Geometry: final body of the model. Coordinates: model frame, mm. A direction names the side the tool comes from. Give positions to 0.01 mm unless a question says otherwise; leave off trailing zeros. Order: outer loops, then holes, each group sorted by start corner. A loop starts at its lowest first (then second) coordinate and runs counter-clockwise, first axis right, second up. Notation, with made-up numbers: (20.25, 42) - (49.25, 42) arc R28 ccw to (49.25, 78) - close; hole circle Ø1 at (-17, 19). An arc over 180 degrees is marked (long way). One line per item, written item: value.
```python
from build123d import *

# Parameters (mm, degrees)
F0_W      = 38.1
F0_H      = 38.1
F1_DEPTH  = 38.1
F6_DEPTH  = 76.2
F8_DEPTH  = 38.1
F9_W      = 25.4
F9_H      = 7.62
F10_DEPTH = 38.1


with BuildPart() as f1:
    # F0 (on Front) → F1 (new body)
    with BuildSketch(Plane.XZ):
        with Locations((-19.05, 19.05)):
            Rectangle(F0_W, F0_H)
    extrude(amount=F1_DEPTH)

    # F5 (on offset) → F6 (cut)
    with BuildSketch(Plane.YZ.offset(38.1)):
        Polygon((-31.75, 0), (-38.1, 38.1), (-38.1, 0), align=None)
        Polygon((-11.43, 16.014082), (-6.35, 38.1), (-31.75, 38.1), (-26.67, 15.896983), (-21.59, 28.575), (-16.51, 28.575), align=None)
        Polygon((-25.4, 0), (-12.7, 0), (-19.05, 15.875), align=None)
        Polygon((-6.35, 0), (0, 0), (0, 38.1), align=None)
    extrude(amount=-F6_DEPTH, mode=Mode.SUBTRACT)

    # F7 (on offset) → F8 (cut)
    with BuildSketch(Plane.XZ.offset(38.1)):
        Polygon((-31.75, 38.1), (-38.1, 38.1), (-38.1, 0), align=None)
        Polygon((-12.7, 38.1), (-25.4, 38.1), (-19.05, 22.225), align=None)
        Polygon((0, 38.1), (-6.35, 38.1), (0, 0), align=None)
        Polygon((-26.67, 22.177041), (-31.75, -0.026754), (-6.350338, -0.133766), (-11.430338, 22.112834), (-16.510338, 9.525), (-21.590338, 9.525), align=None)
    extrude(amount=-F8_DEPTH, mode=Mode.SUBTRACT)

    # F9 (on offset) → F10 (cut)
    with BuildSketch(Plane.XY.offset(38.1)):
        with Locations((-12.7, -11.43)):
            Rectangle(F9_W, F9_H)
        with Locations((-25.4, -26.67)):
            Rectangle(F9_W, F9_H)
    extrude(amount=-F10_DEPTH, mode=Mode.SUBTRACT)


solid = f1.part
```
1) Mould query, pull axis X, two halves, no side actions, for faces 1 (the face through (-12.7, -30, 23)), 2 (the face through (-20.338, -19.103, 25.444)), 3 (the face through (-22.27, -33.5, 30.27)), 4 (the face through (-26.999, -22.234, 26.968)). Classes: released by +X, released by -X, zero draft, split by the parting line, or undercut.
Answers below:
face 1: released by -X
face 2: undercut
face 3: undercut
face 4: zero draft
2) Section B-B, the plane z = 23.5. Count the separate pieces of the cut face and the enclosed holes in it, then the cut area to 3 significant figures.
Answers below:
separate pieces: 6
enclosed holes: 0
area: 576 mm^2
3) Set-up query: faces 5 (the face through (-27.861, -31.124, 35.363)), 6 (the face through (-19, -20, 13.5)), 7 (the face through (-9.43, -5.73, 13.36)). Return all of +Z, -Z, +X, -X, +Y, -Y with unobstructed straight access to the full face (end or side cutting, diameter ignored); none if empty.
Answers below:
face 5: +Z, +X, -X
face 6: -Z, +X, -X
face 7: -Z, +Y, -Y
4) First-contact query: pin 1 (12.5 mm diameter, centred on x = -12, z = 22, fed in from -Y); pin 2 (2.5 mm diameter, centred on y = -28.5, z = 23, fed in from -X); pin 3 (3 mm diameter, centred on y = -21, z = 24.5, fed in from +X); pin 4 (5 mm diameter, centred on y = -20, z = 6, fed in from -X). Flat tips, straight axial feed; report the tip coordinate or a pass-through.
Answers below:
pin 1: y = -36.46
pin 2: x = -12.7
pin 3: x = -3.83
pin 4: through
5) Section A-A, the plane z = 35. Return loops of the section in (x, y).
Answers below:
outline: (-32.27, -37.58) - (-24.16, -37.58) - (-24.16, -31.04) - (-32.27, -31.04) - close; (-32.27, -7.06) - (-24.16, -7.06) - (-24.16, -0.52) - (-32.27, -0.52) - close; (-13.94, -37.58) - (-5.83, -37.58) - (-5.83, -31.04) - (-13.94, -31.04) - close; (-13.94, -7.06) - (-5.83, -7.06) - (-5.83, -0.52) - (-13.94, -0.52) - close
6) Material intervals for line 1 along X through (y, z) = (-4.5, 16.5); line 2 along Y through (x, z) = (-23, 21); line 3 along Y through (x, z) = (-24, 24), sorted ascending.
Answers below:
line 1: -35.35 to -27.97, -24.39 to -13.7, -10.15 to -2.75
line 2: -35.25 to -30.48, -22.86 to -15.24, -7.62 to -2.85
line 3: -35.75 to -30.48, -22.86 to -15.24, -7.62 to -2.35
